Build history of the part. All positions in model axes, mm. A direction names the side the tool comes from. Give positions to 0.01 mm unless a question says otherwise; leave off trailing zeros. Loops run counter-clockwise (first coordinate to the right, second up) from the corner with the lowest first, then second, coordinate; pieces in that order, holes last. Notation, with made-up numbers: (-5, 0.25) -> (7, 0.25) arc R21 ccw to (7, 27.25) -> close; hole circle Ø11 at (45, 73.5). An arc over 180 degrees is marked (long way). One line per question, with ' | ' between items. Start each with the question number.
(1) Drill centre lines: L1, parallel to Y at x = 0.45, z = 29; L2, parallel to Z at x = -1.65, y = -0.25; L3, parallel to Y at x = -0.05, z = 9. Where is each one in solid material? Low to high. Write a range as from..to.
(2) 3-axis set-ups, long thin cutter, end or side, ignore diameter. For faces 4 (the face through (-0.54, -2.44, 35.28)), 5 (the face through (0, 0, 35)): which of +Z, -Z, +X, -X, +Y, -Y reach the whole face in a straight line?
(3) Flat gauge pins, fed straight in: pin 1 Ø1 at (x, y) = (0, 0) entering from +Z; pin 2 Ø2 at (y, z) = (1, 20) entering from +X; pin 3 Ø1.5 at (x, z) = (1, 26.5) entering from -Y. Where does each tip first touch, or does it go through?
(4) Slice it at A-A, the plane z = 28. Write the cut outline in (x, y), then the cut area to 3 significant figures.
(5) Mould opens along Y. For faces 1 (the face through (1.2, -0.9, 36.3)), 2 (the face through (0, -2, 34)), 3 (the face through (-1.5, 0.07, 16.89)) say: pulls with the +Y half, pulls with the -Y half, needs draft (parallel to the pull), parting line crosses it, or undercut.
```python
from build123d import *

# Parameters (mm, degrees)
SKETCH1_R           = 1.5
BOSS_EXTRUDE1_DEPTH = 34
SKETCH2_R           = 2.5
BOSS_EXTRUDE2_DEPTH = 3
CUT_EXTRUDE1_DEPTH  = 2
FILLET1_R           = 0.4
CHAMFER1_SIZE       = 0.25
FILLET2_R           = 0.5


with BuildPart() as part:
    # Sketch1 → Boss-Extrude1 (new body)
    with BuildSketch(Plane.XY):
        Circle(SKETCH1_R)
    extrude(amount=BOSS_EXTRUDE1_DEPTH)

    # Sketch2 → Boss-Extrude2 (add)
    with BuildSketch(Plane.XY.offset(34)):
        Circle(SKETCH2_R)
    extrude(amount=BOSS_EXTRUDE2_DEPTH)

    # Sketch3 → Cut-Extrude1 (cut)
    with BuildSketch(Plane.XY.offset(37)):
        Polygon((1.72759491, -0.124160484), (0.971323588, 1.434060838), (-0.756271322, 1.558221322), (-1.72759491, 0.124160484), (-0.971323588, -1.434060838), (0.756271322, -1.558221322), align=None)
    extrude(amount=-CUT_EXTRUDE1_DEPTH, mode=Mode.SUBTRACT)

    # Fillet1
    fillet1_edges = [part.edges().sort_by_distance(p)[0] for p in [
        (-2.5, 0, 37),
    ]]
    fillet(fillet1_edges, radius=FILLET1_R)

    # Chamfer1
    chamfer1_edges = [part.edges().sort_by_distance(p)[0] for p in [
        (-1.5, 0, 0),
    ]]
    chamfer(chamfer1_edges, length=CHAMFER1_SIZE)

    # Fillet2
    fillet2_edges = [part.edges().sort_by_distance(p)[0] for p in [
        (1.241933116, -0.841190903, 35),
        (-0.107526133, -1.49614108, 35),
        (-1.349459249, -0.654950177, 35),
        (-1.241933116, 0.841190903, 35),
        (0.107526133, 1.49614108, 35),
        (1.349459249, 0.654950177, 35),
    ]]
    fillet(fillet2_edges, radius=FILLET2_R)


solid = part.part
```
Final values:
1) L1: -1.43..1.43 | L2: 34..37 | L3: -1.5..1.5
2) face 4: +Z, -Z | face 5: +Z
3) pin 1: z = 35 | pin 2: x = 1.5 | pin 3: y = -1.48
4) outline: circle Ø3 at (0, 0) | area: 7.07 mm2
5) face 1: undercut | face 2: needs draft | face 3: parting line crosses it
